from build123d import *

# Parameters (mm, degrees)
SKETCH_1_R      = 7
EXTRUDE_1_DEPTH = 45
EXTRUDE_2_DEPTH = 7
SKETCH_7_R      = 4
EXTRUDE_3_DEPTH = 135
SKETCH_8_R      = 2
EXTRUDE_4_DEPTH = 3


with BuildPart() as part:
    # 草图1 → 凸台-拉伸1 (new body)
    with BuildSketch(Plane.XY):
        with Locations(Location((-86.606649797, -63.783530386, 0), (0, 0, 180))):
            Circle(SKETCH_1_R)
    extrude(amount=EXTRUDE_1_DEPTH)

    # 草图3 → 凸台-拉伸2 (add)
    with BuildSketch(Plane(origin=(0, 0, 0), x_dir=(-1, 0, 0), z_dir=(0, 0, -1))):
        with BuildLine():
            Line((87.955581339, -67.549215409), (12.641880873, -94.52784625))
            ThreePointArc((12.641880873, -94.52784625), (7.527264308, -92.111092769), (9.944017789, -86.996476204))
            Line((9.944017789, -86.996476204), (85.257718255, -60.017845362))
            ThreePointArc((85.257718255, -60.017845362), (90.37233482, -62.434598843), (87.955581339, -67.549215409))
        make_face()
    extrude(amount=-EXTRUDE_2_DEPTH)

    # 草图7 → 凸台-拉伸3 (add)
    with BuildSketch(Plane.XY.offset(7)):
        with Locations(Location((-11.292949331, -90.762161227, 0), (0, 0, 250.291624105))):
            Circle(SKETCH_7_R)
    extrude(amount=EXTRUDE_3_DEPTH)

    # 草图8 → 凸台-拉伸4 (add)
    with BuildSketch(Plane.XY.offset(142)):
        Polygon((-11.882983583, -74.617445076), (16.359654092, -84.734431642), (6.242667526, -112.977069317), (-21.999970149, -102.860082751), align=None)
        with Locations((-8.862041731, -81.010715783)):
            Circle(SKETCH_8_R, mode=Mode.SUBTRACT)
        with Locations((9.966383385, -87.755373494)):
            Circle(SKETCH_8_R, mode=Mode.SUBTRACT)
        with Locations((-15.606699442, -99.8391409)):
            Circle(SKETCH_8_R, mode=Mode.SUBTRACT)
        with Locations((3.221725675, -106.58379861)):
            Circle(SKETCH_8_R, mode=Mode.SUBTRACT)
        with Locations((-2.820158028, -93.797257197)):
            Circle(SKETCH_8_R, mode=Mode.SUBTRACT)
    extrude(amount=EXTRUDE_4_DEPTH)


solid = part.part
The model under review builds one solid part; all positions refer to its coordinate system, in mm. A direction names the side the tool comes from. Round coordinates to 2 decimals unless told otherwise and drop trailing zeros. Order: outer loops, then holes, each group sorted by start corner. A loop starts at its lowest first (then second) coordinate and runs counter-clockwise, first axis right, second up. Notation, with made-up numbers: (68, 27) -> (84, 27) arc R25 cw to (84, 43) -> close; hole circle Ø2 at (25.25, 48). An arc over 180 degrees is marked (long way). Write item = value, one per line. Start each with the question number.
Item 1: Consider section D-D on x = -46.5. Write out the cut boundary in (y, z), plus the area to 3 significant figures.
Item 2: For faces 5 (the face through (-3.25, -95.75, 143.48)), 6 (the face through (-93.07, -61.1, 22.18)), list the 3-axis set-ups (+Z, -Z, +X, -X, +Y, -Y) from which the entire face can be reached by the end or side of a thin tool; tool diameter is ignored.
Item 3: Mouldability with a two-part tool opening along X and no side actions: class faces 1 (the face through (-17, -88.9, 143.5)), 2 (the face through (11.37, -98.66, 143.48)), 3 (the face through (-16, -101.8, 143.5)), 4 (the face through (-46, -78, 7)) as released by +X, released by -X, zero draft, split by the parting line, or undercut.
Item 4: Consider section C-C on z = 116. Write out the cut boundary in (x, y), plus the area to 3 significant figures.
Item 5: Clearance check with flat-ended pins moving along their axes: pin 1 Ø5 at (x, y) = (3.22, -106.58) entering from -Z; pin 2 Ø3 at (x, y) = (-2.82, -93.8) entering from -Z; pin 3 Ø11 at (x, y) = (-88, -64) entering from +Z; pin 4 Ø5 at (x, z) = (-80, 40.5) entering from +Y. State where each tip first meets the part, or that it passes through.
Item 6: Consider section B-B on z = 22.5. Write out the cut boundary in (x, y).
Item 7: Consider section A-A on y = -67.5. Write out the cut boundary in (x, z), plus the area to 3 significant figures.
Item 8: For line 1 along Z through (x, y) = (-15, -84); line 2 along Z through (x, y) = (-56, -76.5); line 3 along X through (y, z) = (-68, 20), list the stretches that pass through material, from the lowest coordinate up.
Conclusion:
q1.outline = (-82.4, 0) -> (-73.9, 0) -> (-73.9, 7) -> (-82.4, 7) -> close
q1.area = 59.5 mm2
q2.face_5 = +Z, -Z
q2.face_6 = +Z
q3.face_1 = released by -X
q3.face_2 = released by +X
q3.face_3 = undercut
q3.face_4 = zero draft
q4.outline = circle Ø8 at (-11.29, -90.76)
q4.area = 50.3 mm2
q5.pin_1 = 142
q5.pin_2 = through
q5.pin_3 = 45
q5.pin_4 = -58.11
q6.outline = circle Ø14 at (-86.61, -63.78); circle Ø8 at (-11.29, -90.76)
q7.outline = (-92.54, 0) -> (-64.37, 0) -> (-64.37, 7) -> (-80.67, 7) -> (-80.67, 45) -> (-92.54, 45) -> close
q7.area = 648 mm2
q8.line_1 = 142 to 145
q8.line_2 = 0 to 7
q8.line_3 = -92.19 to -81.02
